```python
from build123d import *

# Parameters (mm, degrees)
EXTRUDE_1_DEPTH     = 332
SKETCH_2_R          = 3.25
CUT_EXTRUDE_1_DEPTH = 5
SKETCH_3_R          = 5
CUT_EXTRUDE_2_DEPTH = 5
SKETCH_4_W          = 26.179083289
SKETCH_4_H          = 3.25731829
CUT_EXTRUDE_3_DEPTH = 10
SKETCH_5_R          = 1.75
CUT_EXTRUDE_4_DEPTH = 2.5
CHAMFER_1_SIZE      = 1.5


with BuildPart() as part:
    # Эскиз1 → Вытянуть1 (new body)
    with BuildSketch(Plane.XY):
        with BuildLine():
            Line((-1, -68), (-1, 104))
            ThreePointArc((-1, 104), (0.171572875, 106.828427125), (3, 108))
            Line((3, 108), (24, 108))
            Line((24, 108), (24, 106))
            Line((24, 106), (3, 106))
            ThreePointArc((3, 106), (1.585786438, 105.414213562), (1, 104))
            Line((1, 104), (1, -68))
            ThreePointArc((1, -68), (-0.171572875, -70.828427125), (-3, -72))
            Line((-3, -72), (-44, -72))
            Line((-44, -72), (-44, -70))
            Line((-44, -70), (-3, -70))
            ThreePointArc((-3, -70), (-1.585786438, -69.414213562), (-1, -68))
        make_face()
    extrude(amount=EXTRUDE_1_DEPTH)

    # Эскиз2 → Вырез-Вытянуть1 (cut)
    with BuildSketch(Plane.ZY.offset(1)):
        with Locations((31, -38)):
            Circle(SKETCH_2_R)
        with Locations((121, -38)):
            Circle(SKETCH_2_R)
        with Locations((211, -38)):
            Circle(SKETCH_2_R)
        with Locations((301, -38)):
            Circle(SKETCH_2_R)
    extrude(amount=-CUT_EXTRUDE_1_DEPTH, mode=Mode.SUBTRACT)

    # Эскиз3 → Вырез-Вытянуть2 (cut)
    with BuildSketch(Plane(origin=(0, -70, 0), x_dir=(1, 0, 0), z_dir=(0, 1, 0))):
        with Locations(Location((-24, -18.5, 0), (0, 0, 270))):
            Circle(SKETCH_3_R)
        with Locations(Location((-24, -313.5, 0), (0, 0, 270))):
            Circle(SKETCH_3_R)
    extrude(amount=-CUT_EXTRUDE_2_DEPTH, mode=Mode.SUBTRACT)

    # Эскиз4 → Вырез-Вытянуть3 (cut)
    with BuildSketch(Plane(origin=(0, 108, 0), x_dir=(1, 0, 0), z_dir=(0, 1, 0))):
        with Locations((16.089541645, 0.628659145)):
            Rectangle(SKETCH_4_W, SKETCH_4_H)
        with Locations((16.089541645, -332.628659145)):
            Rectangle(SKETCH_4_W, SKETCH_4_H)
    extrude(amount=-CUT_EXTRUDE_3_DEPTH, mode=Mode.SUBTRACT)

    # Эскиз5 → Вырез-Вытянуть4 (cut)
    with BuildSketch(Plane.ZY.offset(1)):
        with Locations(Location((5.7, 95, 0), (0, 0, 270))):
            Circle(SKETCH_5_R)
        with Locations(Location((326.3, 95, 0), (0, 0, 270))):
            Circle(SKETCH_5_R)
    extrude(amount=-CUT_EXTRUDE_4_DEPTH, mode=Mode.SUBTRACT)

    # Фаска1
    chamfer_1_edges = [part.edges().sort_by_distance(p)[0] for p in [
        (-1, 96.75, 326.3),
        (-1, 96.75, 5.7),
    ]]
    chamfer(chamfer_1_edges, length=CHAMFER_1_SIZE)


solid = part.part
```
Read the model definition and answer for the solid it produces. Units are mm, in the model's axes. A direction names the side the tool comes from. Round coordinates to 2 decimals unless told otherwise and drop trailing zeros. Loops run counter-clockwise (first coordinate to the right, second up) from the corner with the lowest first, then second, coordinate; pieces in that order, holes last. Notation, with made-up numbers: (-20.5, 0) -> (12.5, 0) arc R32 ccw to (12.5, 26) -> close; hole circle Ø10 at (57.25, 7). An arc over 180 degrees is marked (long way). One line per item, written item: value.
1) The mould has two halves that part along Y. Classify faces 1 (the face through (-0.014, -40.883, 32.5)), 2 (the face through (-28.88, -70.99, 17.42)), 3 (the face through (-0.014, -39.245, 214.002)), 4 (the face through (14, 106, 164)): pulls with the +Y half, pulls with the -Y half, needs draft (parallel to the pull), parting line crosses it, or undercut.
Answer list:
face 1: undercut
face 2: needs draft
face 3: undercut
face 4: pulls with the -Y half
2) A cutting plane is placed at A-A (x = -24). Determine the outline of the cut face in (y, z).
Answer list:
outline: (-72, 0) -> (-70, 0) -> (-70, 13.5) -> (-72, 13.5) -> close; (-72, 23.5) -> (-70, 23.5) -> (-70, 308.5) -> (-72, 308.5) -> close; (-72, 318.5) -> (-70, 318.5) -> (-70, 332) -> (-72, 332) -> close
3) A cutting plane is placed at C-C (z = 222). Determine the outline of the cut face in (x, y).
Answer list:
outline: (-44, -72) -> (-3, -72) arc R4 ccw to (1, -68) -> (1, 104) arc R2 cw to (3, 106) -> (24, 106) -> (24, 108) -> (3, 108) arc R4 ccw to (-1, 104) -> (-1, -68) arc R2 cw to (-3, -70) -> (-44, -70) -> close
4) For faces 5 (the face through (-0.014, -40.883, 122.5)), 6 (the face through (-24, -70, 164)), 7 (the face through (1, 19, 164)), determine the directions among +Z, -Z, +X, -X, +Y, -Y from which every point of the face is accessible in a straight line to the end or side of a thin tool.
Answer list:
face 5: +X, -X
face 6: +Z, -Z, -X, +Y
face 7: +Z, -Z, +X, -Y
5) Flat-ended cylindrical pins translate along their axes: P1, Ø7.5, axis at y = -38, z = 301, coming from the -X side; P2, Ø2, axis at y = 95, z = 326.3, coming from the +X side; P3, Ø11.5, axis at x = -24, z = 18.5, coming from the +Y side; P4, Ø10.5, axis at x = 8.5, z = 196.5, coming from the -Y side. Find the tip coordinate at first contact, or state that the pin passes through.
Answer list:
P1: stops at x = -1
P2: passes through
P3: stops at y = -70
P4: stops at y = 106
6) Consider L1, parallel to Y at x = -31, z = 212.5; L2, parallel to X at y = -20, z = 53.5; L3, parallel to Y at x = 0.05, z = 211. Determine where each line is inside the solid, lowest interval first. Write a range as [from, to].
Answer list:
L1: y = [-72, -70]
L2: x = [-1, 1]
L3: y = [-70.59, -41.25], [-34.75, 106.7]
7) A cutting plane is placed at D-D (y = 53). Determine the outline of the cut face in (x, z).
Answer list:
outline: (-1, 0) -> (1, 0) -> (1, 332) -> (-1, 332) -> close
8) A cutting plane is placed at B-B (z = 121). Determine the outline of the cut face in (x, y).
Answer list:
outline: (-44, -72) -> (-3, -72) arc R4 ccw to (1, -68) -> (1, -41.25) -> (-1, -41.25) -> (-1, -68) arc R2 cw to (-3, -70) -> (-44, -70) -> close; (-1, -34.75) -> (1, -34.75) -> (1, 104) arc R2 cw to (3, 106) -> (24, 106) -> (24, 108) -> (3, 108) arc R4 ccw to (-1, 104) -> close
